```python
from build123d import *

# Parameters (mm, degrees)
F0_W     = 36.92906
F0_H     = 100.3808
F1_DEPTH = 2.54
F2_W     = 36.92906
F2_H     = 31.99892
F3_DEPTH = 15.24
F4_T     = -2.54
F5_W     = 31.84906
F5_H     = 26.91892
F6_DEPTH = 2.54


# Not quite as in the source:
# - a shell that OpenCascade refuses in one call is made with other operations: the cavity is built on its own and cut out


with BuildPart() as f1:
    # F0 (on Front) → F1 (new body)
    with BuildSketch(Plane.XZ):
        with Locations((-3.5625953953, 0.4117265198)):
            Rectangle(F0_W, F0_H)
    extrude(amount=F1_DEPTH)

    # F2 (on face) → F3 (join)
    with BuildSketch(Plane.XZ.offset(2.54)):
        with Locations((-3.5625953953, 0.3964865198)):
            Rectangle(F2_W, F2_H)
    extrude(amount=-F3_DEPTH)

    # F4: a shell. OpenCascade refuses it in one call, so the cavity is built on its own and cut out:
    # the body offset inwards by the wall thickness, plus a prism from it out through each open face.
    f4_core = offset(f1.part, amount=F4_T, kind=Kind.INTERSECTION, mode=Mode.PRIVATE)
    f4_exits = [f4_core.faces().sort_by_distance(p)[0] for p in [
        (-3.562595, 5.08, 13.855947),
    ]]
    add(f4_core, mode=Mode.SUBTRACT)
    extrude(f4_exits, amount=-F4_T, mode=Mode.SUBTRACT)

    # F5 (on face) → F6 (cut, through all)
    with BuildSketch(Plane(origin=(0, 12.7, 0), x_dir=(-1, 0, 0), z_dir=(0, 1, 0))):
        with Locations((3.5625953953, 0.3964865198)):
            Rectangle(F5_W, F5_H)
    extrude(amount=-F6_DEPTH, mode=Mode.SUBTRACT)


solid = f1.part
```
The listing builds one solid part. Answer for the finished solid, in the listing's coordinates (mm). A direction names the side the tool comes from. Give positions to 0.01 mm unless a question says otherwise; leave off trailing zeros. Loops run counter-clockwise (first coordinate to the right, second up) from the corner with the lowest first, then second, coordinate; pieces in that order, holes last. Notation, with made-up numbers: M 51.25,55.5 L 82.25,55.5 A22 ccw 82.25,63.5 Z; hole C 64,1 d8. An arc over 180 degrees is marked long. One line per item, written item: value.
1. For a pull along Z with two mould halves and no side action, classify faces 1 (the face through (-19.487, 6, 1)), 2 (the face through (-4, 12.7, -14)), 3 (the face through (-4, -1, -49.779)) as pulls with the +Z half, pulls with the -Z half, needs draft (parallel to the pull), parting line crosses it, or undercut.
Found:
face 1: undercut
face 2: needs draft
face 3: pulls with the -Z half
2. Section B-B on y = 2.5 is taken. Determine the outline of the cut face in (x, z), plus the area to 3 significant figures.
Found:
outline: M -22.03,-15.6 L 14.9,-15.6 L 14.9,16.4 L 12.36,16.4 L 12.36,-13.06 L -19.49,-13.06 L -19.49,16.4 L -22.03,16.4 Z
area: 243 mm^2
3. For faces 4 (the face through (-4, 10.16, 15)), 5 (the face through (-4, -2.54, 1)), 6 (the face through (-4, 6, -13.063)), 7 (the face through (-4, 6, -15.603)), 8 (the face through (-3.8, 10.5, 16.396)), determine the directions among +Z, -Z, +X, -X, +Y, -Y from which every point of the face is accessible in a straight line to the end or side of a thin tool.
Found:
face 4: +Z
face 5: +Z, -Z, +X, -X, -Y
face 6: +Y
face 7: -Z, +X, -X, +Y
face 8: +Z, +X, -X, +Y
4. Section A-A on x = 8 is taken. Determine the outline of the cut face in (y, z), plus the area to 3 significant figures.
Found:
outline: M -2.54,-49.78 L 0,-49.78 L 0,-15.6 L 12.7,-15.6 L 12.7,-13.06 L 0,-13.06 L 0,50.6 L -2.54,50.6 Z; M 10.16,13.86 L 12.7,13.86 L 12.7,16.4 L 10.16,16.4 Z
area: 294 mm^2
5. Section C-C on z = 6 is taken. Determine the outline of the cut face in (x, y).
Found:
outline: M -22.03,-2.54 L 14.9,-2.54 L 14.9,12.7 L 12.36,12.7 L 12.36,0 L -19.49,0 L -19.49,12.7 L -22.03,12.7 Z
6. Section D-D on y = 11.5 is taken. Determine the outline of the cut face in (x, z).
Found:
outline: M -22.03,-15.6 L 14.9,-15.6 L 14.9,16.4 L -22.03,16.4 Z; hole M -19.49,-13.06 L 12.36,-13.06 L 12.36,13.86 L -19.49,13.86 Z
7. Each of these flat-tipped pins is pushed along its axis until it touches: P1, Ø1.5, axis at x = -5.5, y = 7, coming from the +Z side; P2, Ø5, axis at y = 3.5, z = 20.5, coming from the -X side; P3, Ø4, axis at x = -11.5, y = 5.5, coming from the -Z side. Where does it stop, or does it pass through?
Found:
P1: z = -13.06
P2: through
P3: z = -15.6
8. Find the intervals of material crossed by probe 1 along Y at (x, z) = (-10.5, 14.5); probe 2 along X at (y, z) = (7, 3.5); probe 3 along Z at (x, y) = (8.5, 10.25), in increasing order.
Found:
probe 1: -2.54 to 0, 10.16 to 12.7
probe 2: -22.03 to -19.49, 12.36 to 14.9
probe 3: -15.6 to -13.06, 13.86 to 16.4
